Part model, mm, in its own coordinate system. A direction names the side the tool comes from. Give positions to 0.01 mm unless a question says otherwise; leave off trailing zeros. Loops run counter-clockwise (first coordinate to the right, second up) from the corner with the lowest first, then second, coordinate; pieces in that order, holes last. Notation, with made-up numbers: (74.5, 72) -> (79.5, 72) arc R26 cw to (79.5, 109) -> close; hole circle Ø1 at (77.25, -32). An arc over 180 degrees is marked (long way). Write item = value, one per line.
Autodesk Inventor part; units mm, degrees
ref_plane "YZ Plane" through (0, 0, 0) normal (1, 0, 0) x (0, 1, 0)
ref_plane "XZ Plane" through (0, 0, 0) normal (0, 1, 0) x (-1, 0, 0)
ref_plane "XY Plane" through (0, 0, 0) normal (0, 0, 1) x (1, 0, 0)
sketch "スケッチ1" plane through (0, 0, 0) normal (0, 1, 0) x (-1, 0, 0)
  arc A0 (99.4141, -32.927) -> (304.2493, 7.0592) centre (88.5018, 567.6156) ccw
  arc A1 (73.8469, -32.6347) -> (99.4141, -32.927) centre (91.566, 398.982) ccw
  arc A2 (27.3573, -24.3709) -> (73.8469, -32.6347) centre (81.048, 142.776) ccw
  arc A3 (0.844, -11.3484) -> (27.3573, -24.3709) centre (58.458, 72.45) ccw
  arc A4 (-6.1834, -4.5246) -> (0.844, -11.3484) centre (17.4, 12.732) ccw
  arc A5 (-1.3535, 7.5415) -> (-6.1834, -4.5246) centre (0, 0) ccw
  arc A6 (18.2937, 9.3227) -> (-1.3535, 7.5415) centre (18.66, -103.968) ccw
  arc A7 (85.069, 6.346) -> (18.2937, 9.3227) centre (20.556, -690.396) ccw
  arc A8 (85.069, 6.346) -> (126.1777, 2.6065) centre (1264.674, 12746.1) ccw
  arc A9 (126.1777, 2.6065) -> (203.1141, -0.6229) centre (198.864, 816.2039) ccw
  arc A10 (203.1141, -0.6229) -> (304.2493, 7.0592) centre (199.374, 718.188) ccw
  circle A11 centre (20, -2.2582) radius 6
  circle A12 centre (130, -14.678) radius 6
extrude "押し出し1" add sketch "スケッチ1" along normal mid plane 225 contours A1 A2 A3 A4 A5 A6 A7 A8 A9 A10 A0 | A11 | A12
shell "シェル1" thickness 3 outward yes removed faces 2 at (-113.7457, 112.5, -20.2414) at (-113.7457, -112.5, -20.2414)
properties part number "GFRP_ms"
1) Slice it at B-B, the plane z = -21. List the corners of the cut face in (x, y), and give its area (3 significant figures).
Resolved:
outline = (-222.35, -112.5) -> (-208.09, -112.5) -> (-208.09, 112.5) -> (-222.35, 112.5) -> close; (-18.35, -112.5) -> (-11.26, -112.5) -> (-11.26, 112.5) -> (-18.35, 112.5) -> close
area = 4,800 mm²
2) Drill centre lines: line 1 along Z through (x, y) = (-36.5, -100.5); line 2 along Z through (x, y) = (-61.5, 48.5). Where is each one in solid material? Low to high. Write a range as [from, to].
Resolved:
line_1 = [-30.14, -27.04], [9.14, 12.15]
line_2 = [-34.71, -31.69], [8.13, 11.13]
3) Which spindle directions (+Z, -Z, +X, -X, +Y, -Y) get a long thin tool onto all of the face, cutting with end or side? Do faces 1 (the face through (-164.197, 1.575, 3.105)), 2 (the face through (-8.569, 1.575, 8.873)), 3 (the face through (-8.3, 1.58, 11.86)). Say none if no direction does.
Resolved:
face_1 = +Z, +Y, -Y
face_2 = +Y, -Y
face_3 = +Z, +X, +Y, -Y
4) Drop flat-ended pins along their axis: P1, Ø6, axis at x = -283.5, y = -31, coming from the -Z side; P2, Ø1.5, axis at x = -205, y = -23, coming from the -Z side; P3, Ø1.5, axis at y = -57, z = 7.5, coming from the -X side. Give the stop position or say it passes through.
Resolved:
P1 = -4.68
P2 = -24.82
P3 = -315.42
5) Pull direction Z, two halves, no side cores. Call faces 4 (the face through (-52.32, 1.58, 11.61)), 5 (the face through (-49.997, 1.575, -30.015)), 6 (the face through (9.84, 1.58, 4.1)): pulls with the +Z half, pulls with the -Z half, needs draft (parallel to the pull), parting line crosses it, or undercut.
Resolved:
face_4 = pulls with the +Z half
face_5 = undercut
face_6 = parting line crosses it
6) Slice it at A-A, the plane y = 5.5. List the corners of the cut face in (x, z).
Resolved:
outline = (-330, 14.39) arc R603.64 ccw to (-99.47, -35.93) arc R435.03 ccw to (-73.72, -35.63) arc R178.56 ccw to (-26.44, -27.23) arc R104.69 ccw to (0.86, -13.82) arc R32.22 ccw to (8.6, -6.3) arc R10.66 ccw to (1.88, 10.49) arc R116.29 ccw to (-18.28, 12.32) arc R702.73 ccw to (-85.35, 9.33) arc R12798.36 cw to (-126.44, 5.59) arc R813.85 cw to (-203.1, 2.38) arc R715.81 cw to start; hole (-304.25, 7.06) arc R600.64 ccw to (-99.41, -32.93) arc R432.03 ccw to (-73.85, -32.63) arc R175.56 ccw to (-27.36, -24.37) arc R101.69 ccw to (-0.84, -11.35) arc R29.22 ccw to (6.18, -4.52) arc R7.66 ccw to (1.35, 7.54) arc R113.29 ccw to (-18.29, 9.32) arc R699.73 ccw to (-85.07, 6.35) arc R12801.36 cw to (-126.18, 2.61) arc R816.85 cw to (-203.11, -0.62) arc R718.81 cw to start
